Geometry: final body of the model. Coordinates: model frame, mm. Face numbers are marked on the shaded views. A direction names the side the tool comes from. Round coordinates to 2 decimals unless told otherwise and drop trailing zeros. Write each loop counter-clockwise with the first axis right and the second up, starting at its lowest first coordinate (ties: lowest second). Pieces come first, ordered by that corner, then holes. Notation, with made-up numbers: M -34,13 L 13,13 A19 ccw 13,22 Z; hole C 80.25,53 d8. An arc over 180 degrees is marked long. Answer as CSV lines item,"result". Start each with the question number.
Q1. Section query A-A on y = 9.75. Output: boundary loops of the cut face in (x, z).
Q2. Section query B-B on z = -4. Output: boundary loops of the cut face in (x, y).
Q3. Section query D-D on y = 22.5. Output: boundary loops of the cut face in (x, z).
Q4. Ray query, probe 1 along Z at (x, y) = (7, 20.5); probe 2 along X at (y, z) = (9.5, 17); probe 3 along Y at (x, z) = (19, -30). Return the intervals inside material, ascending.
Q5. First-contact query: pin 1 (1 mm diameter, centred on x = 26.5, z = 18.5, fed in from +Y); pin 2 (5.5 mm diameter, centred on x = -31, z = 4, fed in from +Y). Flat tips, straight axial feed; report the tip coordinate or a pass-through.
Q6. Reachability of the marked faces 4 and 5 from +Z, -Z, +X, -X, +Y, -Y: full face, straight path, thin tool, end or side. Return the list, or none.
Q7. Section query C-C on x = 1.5. Output: boundary loops of the cut face in (y, z), and give its area (3 significant figures).
Q8. Mould query, pull axis Z, two halves, no side actions, for the marked faces 1, 2 and 3. Classes: pulls with the +Z half, pulls with the -Z half, needs draft (parallel to the pull), parting line crosses it, or undercut.
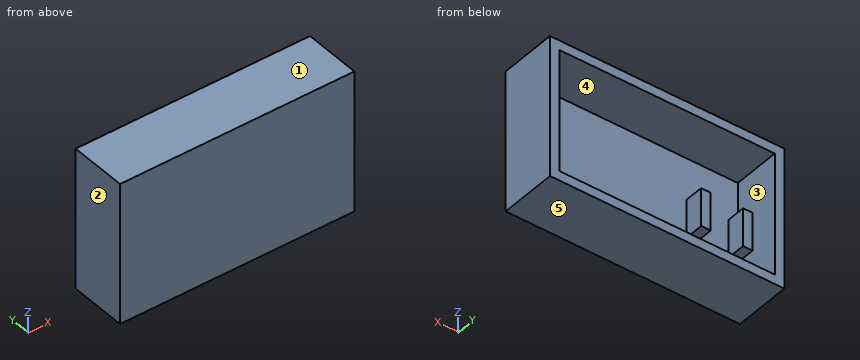
```python
from build123d import *

# Parameters (mm, degrees)
SKETCH1_W           = 123
SKETCH1_H           = 74
BOSS_EXTRUDE1_DEPTH = 30
SKETCH2_W           = 113
SKETCH2_H           = 64
CUT_EXTRUDE1_DEPTH  = 25
BOSS_EXTRUDE2_DEPTH = 10
LPATTERN1_COUNT     = 2
LPATTERN1_PITCH     = 22


with BuildPart() as part:
    # Sketch1 → Boss-Extrude1 (new body)
    with BuildSketch(Plane(origin=(0, 0, 0), x_dir=(1, 0, 0), z_dir=(0, 1, 0))):
        Rectangle(SKETCH1_W, SKETCH1_H)
    extrude(amount=BOSS_EXTRUDE1_DEPTH)

    # Sketch2 → Cut-Extrude1 (cut)
    with BuildSketch(Plane(origin=(0, 30, 0), x_dir=(1, 0, 0), z_dir=(0, 1, 0))):
        Rectangle(SKETCH2_W, SKETCH2_H)
    extrude(amount=-CUT_EXTRUDE1_DEPTH, mode=Mode.SUBTRACT)

    # Sketch4 → Boss-Extrude2 (add)
    with BuildSketch(Plane(origin=(0, 5, 0), x_dir=(1, 0, 0), z_dir=(0, 1, 0))):
        Polygon((-56.5, -10), (-51.5, -10), (-51.5, 10), (-56.5, 10), (-56.5, 0), align=None)
    boss_extrude2 = extrude(amount=BOSS_EXTRUDE2_DEPTH)

    # LPattern1: Boss-Extrude2 ×2
    with Locations(*[(i * LPATTERN1_PITCH, 0, 0) for i in range(1, LPATTERN1_COUNT)]):
        add(boss_extrude2)


solid = part.part
```
Entries:
1,outline,"M -61.5,-37 L 61.5,-37 L 61.5,37 L -61.5,37 Z; M -34.5,-10 L -29.5,-10 L -29.5,10 L -34.5,10 Z; hole M -56.5,-32 L 56.5,-32 L 56.5,32 L -56.5,32 L -56.5,10 L -51.5,10 L -51.5,-10 L -56.5,-10 Z"
2,outline,"M -61.5,0 L 61.5,0 L 61.5,30 L 56.5,30 L 56.5,5 L -29.5,5 L -29.5,15 L -34.5,15 L -34.5,5 L -51.5,5 L -51.5,15 L -56.5,15 L -56.5,30 L -61.5,30 Z"
3,outline,"M -61.5,-37 L 61.5,-37 L 61.5,37 L -61.5,37 Z; hole M -56.5,-32 L 56.5,-32 L 56.5,32 L -56.5,32 Z"
4,probe 1,"z = -37 to -32, 32 to 37"
4,probe 2,"x = -61.5 to -56.5, 56.5 to 61.5"
4,probe 3,"y = 0 to 5"
5,pin 1,"stops at y = 5"
5,pin 2,"stops at y = 15"
6,face 4,"+Y"
6,face 5,"-Z, +X, -X, +Y, -Y"
7,outline,"M 0,-37 L 30,-37 L 30,-32 L 5,-32 L 5,32 L 30,32 L 30,37 L 0,37 Z"
7,area,"620 mm^2"
8,face 1,"pulls with the +Z half"
8,face 2,"needs draft"
8,face 3,"undercut"
